Could you check a few things on this model? Use its own coordinates, in mm. A direction names the side the tool comes from. Give positions to 0.01 mm unless a question says otherwise; leave off trailing zeros. Order: outer loops, then holes, each group sorted by start corner. A loop starts at its lowest first (then second) coordinate and runs counter-clockwise, first axis right, second up. Notation, with made-up numbers: (84.25, -21) -> (122.25, -21) arc R36 cw to (122.25, 17) -> close; hole circle Ø2 at (-27.75, 7). An arc over 180 degrees is marked (long way). One line per item, written item: value.
```python
from build123d import *

# Parameters (mm, degrees)
SKETCH_1_R      = 15
SKETCH_1_R_2    = 8.5
SKETCH_1_R_3    = 10
EXTRUDE_5_DEPTH = 5
EXTRUDE_START   = -3
SKETCH_3_R      = 8.5
EXTRUDE_6_DEPTH = 3
EXTRUDE_8_DEPTH = 50


with BuildPart() as part:
    # 草图1 → 凸台-拉伸5 (new body)
    # profile 1 of 3: a face of its own
    with BuildSketch(Plane(origin=(0, 0, 0), x_dir=(1, 0, 0), z_dir=(0, 1, 0))):
        Circle(SKETCH_1_R)
        with Locations(Location((0, 0, 0), (0, 0, 270))):
            Circle(SKETCH_1_R_2, mode=Mode.SUBTRACT)
    # profile 2 of 3: a face of its own
    with BuildSketch(Plane(origin=(0, 0, 0), x_dir=(1, 0, 0), z_dir=(0, 1, 0))):
        with BuildLine():
            Line((60.699439854, 9.965059042), (1.252835242, 14.947588563))
            ThreePointArc((1.252835242, 14.947588563), (11.040664125, 10.154000969), (15, 0))
            ThreePointArc((15, 0), (11.040664125, -10.154000969), (1.252835242, -14.947588563))
            Line((1.252835242, -14.947588563), (60.699439854, -9.965059042))
            ThreePointArc((60.699439854, -9.965059042), (49.864216359, 0), (60.699439854, 9.965059042))
        make_face()
    # profile 3 of 3: a face of its own
    with BuildSketch(Plane(origin=(0, 0, 0), x_dir=(1, 0, 0), z_dir=(0, 1, 0))):
        with Locations((59.864216359, 0)):
            Circle(SKETCH_1_R_3)
    extrude(amount=EXTRUDE_5_DEPTH)

    # 草图3 → 凸台-拉伸6 (add)
    with BuildSketch(Plane(origin=(0, 5, 0), x_dir=(1, 0, 0), z_dir=(0, 1, 0)).offset(EXTRUDE_START)):
        with Locations(Location((0, 0, 0), (0, 0, 270))):
            Circle(SKETCH_3_R)
    extrude(amount=EXTRUDE_6_DEPTH)

    # 草图4 → 凸台-拉伸8 (add)
    with BuildSketch(Plane(origin=(0, 0, 0), x_dir=(-1, 0, 0), z_dir=(0, -1, 0))):
        Polygon((-64.16134725, -4.724526638), (-64.16134725, 5.275473362), (-54.280111118, 5.275473362), (-56.872098045, 8.381028801), (-64.852894721, 6.995424542), (-67.643324571, -0.608950251), (-62.452957745, -6.827720786), (-54.472161069, -5.442116527), (-54.208841033, -4.724526638), align=None)
        Polygon((-51.681731219, 2.162258266), (-54.16134725, 5.133177977), (-54.16134725, -4.595098362), align=None)
        Polygon((-54.280111118, 5.275473362), (-64.16134725, 5.275473362), (-64.16134725, -4.724526638), (-54.208841033, -4.724526638), (-54.16134725, -4.595098362), (-54.16134725, 5.133177977), align=None)
    extrude(amount=EXTRUDE_8_DEPTH)


solid = part.part
```
1) If I drill on line 1 along X through (y, z) = (1.25, 0); line 2 along Y through (x, z) = (-3, 6.5); line 3 along Y through (x, z) = (14, -3.25), over which ranges is the centre line in solid material (lowest first)?
Answer below:
line 1: x = -15 to -8.5, 8.5 to 69.86
line 2: y = 2 to 5
line 3: y = 0 to 5
2) We'd pull the mould along Z, two halves only. Please class faces 1 (the flat face through (31.39, 2.46, -12.42)), 2 (the cylindrical face through (-15, 2, 0)), 3 (the flat face through (0, 2, 0)): +Z half, -Z half, draft (parallel to the pull), parting line (faces both ways), or undercut.
Answer below:
face 1: -Z half
face 2: parting line
face 3: undercut
3) Suppose I cut it at C-C, the plane z = -3.25. Write out the boundary of the cut face in (x, y), then the cut area to 3 significant figures.
Answer below:
outline: (-14.64, 0) -> (-7.85, 0) -> (-7.85, 2) -> (7.85, 2) -> (7.85, 0) -> (52.59, 0) -> (52.59, -50) -> (66.23, -50) -> (66.23, 0) -> (69.32, 0) -> (69.32, 5) -> (-14.64, 5) -> close
area: 1,070 mm2
4) For P1, Ø9, axis at x = 45.5, z = -1.5, coming from the -Y side; P2, Ø12, axis at x = 57, y = -16.5, coming from the -Z side, each with a flat end and sliding along its axis, tell me the tip position at first contact or that it passes through.
Answer below:
P1: stops at y = 0
P2: stops at z = -8.38
5) Suppose I cut it at B-B, the plane x = 0. Write out the boundary of the cut face in (y, z).
Answer below:
outline: (0, -15) -> (5, -15) -> (5, 15) -> (0, 15) -> (0, 8.5) -> (2, 8.5) -> (2, -8.5) -> (0, -8.5) -> close
6) For faces 4 (the flat face through (58.518, -24.65, 6.145)), 5 (the flat face through (65.084, -24.65, 3.675)), 6 (the flat face through (60.8, -24.6, -7.7)), which set-ups out of +Z, -Z, +X, -X, +Y, -Y let a thin tool reach every point of the face, with its end or its side?
Answer below:
face 4: +Z, -X, -Y
face 5: +Z, +X, -Y
face 6: -Z, +X, -Y
7) Suppose I cut it at A-A, the plane y = -17. Write out the boundary of the cut face in (x, z).
Answer below:
outline: (51.68, -2.16) -> (56.87, -8.38) -> (64.85, -7) -> (67.64, 0.61) -> (62.45, 6.83) -> (54.47, 5.44) -> close
8) Suppose I cut it at D-D, the plane x = 59.5. Write out the boundary of the cut face in (y, z), then the cut area to 3 significant figures.
Answer below:
outline: (-50, -7.92) -> (0, -7.92) -> (0, -10.07) -> (5, -10.07) -> (5, 10.07) -> (0, 10.07) -> (0, 6.32) -> (-50, 6.32) -> close
area: 813 mm2
